For this review, take the finished solid that the model builds, in its own axes (mm). Face numbers are marked on the shaded views. A direction names the side the tool comes from. Round coordinates to 2 decimals unless told otherwise and drop trailing zeros. Write each loop counter-clockwise with the first axis right and the second up, starting at its lowest first coordinate (ties: lowest second). Pieces come first, ordered by that corner, then holes. Notation, with made-up numbers: M 6,58.25 L 20,58.25 A10 cw 20,76.25 Z; hole C -33.5,72.5 d3. An arc over 180 degrees is marked long. Answer in a Markdown table with one row per item.
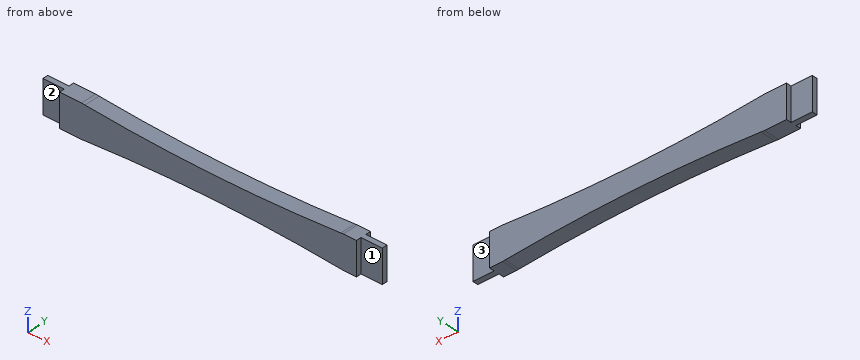
```python
from build123d import *

# Parameters (mm, degrees)
F0_W     = 406.4
F0_H     = 39.6875
F1_DEPTH = 9.525
F2_W     = 25.4
F2_H     = 6.35
F3_DEPTH = 39.6885
F5_DEPTH = 19.051


with BuildPart() as f1:
    # F0 (on Front) → F1 (new body, symmetric)
    with BuildSketch(Plane.XZ):
        Rectangle(F0_W, F0_H)
    extrude(amount=F1_DEPTH, both=True)

    # F2 (on face) → F3 (cut, through all)
    with BuildSketch(Plane.XY.offset(19.84375)):
        with Locations((190.5, -6.35)):
            Rectangle(F2_W, F2_H)
        with Locations((190.5, 6.35)):
            Rectangle(F2_W, F2_H)
        with Locations((-190.5, -6.35)):
            Rectangle(F2_W, F2_H)
        with Locations((-190.5, 6.35)):
            Rectangle(F2_W, F2_H)
    extrude(amount=-F3_DEPTH, mode=Mode.SUBTRACT)

    # F4 (on face) → F5 (cut, through all)
    with BuildSketch(Plane.XZ.offset(9.525)):
        with BuildLine():
            Line((162.1778154521, 19.84375), (-151.4870877189, 19.84375))
            ThreePointArc((-151.4870877189, 19.84375), (-149.3549908007, 19.6719963975), (-147.222705797, 19.5025938249))
            ThreePointArc((-147.222705797, 19.5025938249), (6.0616249582, 13.493882231), (159.3414767794, 19.6157851846))
            ThreePointArc((159.3414767794, 19.6157851846), (160.7596879137, 19.7292475425), (162.1778154521, 19.84375))
        make_face()
        with BuildLine():
            ThreePointArc((-147.222705797, -19.5025938249), (-149.3549908007, -19.6719963975), (-151.4870877189, -19.84375))
            Line((-151.4870877189, -19.84375), (162.1778154521, -19.84375))
            ThreePointArc((162.1778154521, -19.84375), (160.7596879137, -19.7292475425), (159.3414767794, -19.6157851846))
            ThreePointArc((159.3414767794, -19.6157851846), (6.0616249582, -13.493882231), (-147.222705797, -19.5025938249))
        make_face()
    extrude(amount=-F5_DEPTH, mode=Mode.SUBTRACT)


solid = f1.part
```
Q1. Take a section at D-D (x = 103). State the section outline as (y, z) points (3 decimals).
Found:
| item | result |
|---|---|
| outline | M -9.525,-15.953 L 9.525,-15.953 L 9.525,15.953 L -9.525,15.953 Z |
Q2. Insertion check: P1, Ø7, axis at y = -7.5, z = 5, coming from the +X side; P2, Ø12.5, axis at x = -190, z = 0, coming from the +Y side (3 decimals); P3, Ø7.5, axis at x = -192.5, z = -7, coming from the -Y side (3 decimals). Each pin has a flat end and moves straight along its axis. Give the tip position at first contact, or say it passes through.
Found:
| item | result |
|---|---|
| P1 | x = 177.8 |
| P2 | y = 3.175 |
| P3 | y = -3.175 |
Q3. Take a section at C-C (x = -100.5). State the section outline as (y, z) points (3 decimals).
Found:
| item | result |
|---|---|
| outline | M -9.525,-16.383 L 9.525,-16.383 L 9.525,16.383 L -9.525,16.383 Z |
Q4. Take a section at B-B (z = 0). State the section outline as (x, y) points (3 decimals).
Found:
| item | result |
|---|---|
| outline | M -203.2,-3.175 L -177.8,-3.175 L -177.8,-9.525 L 177.8,-9.525 L 177.8,-3.175 L 203.2,-3.175 L 203.2,3.175 L 177.8,3.175 L 177.8,9.525 L -177.8,9.525 L -177.8,3.175 L -203.2,3.175 Z |
Q5. Take a section at A-A (y = 0.25). State the section outline as (x, z) points, then the cut area to 3 significant figures.
Found:
| item | result |
|---|---|
| outline | M -203.2,-19.84 L -151.49,-19.84 A1939.9 cw -147.22,-19.5 A1939.9 cw 159.34,-19.62 A1939.9 cw 162.18,-19.84 L 203.2,-19.84 L 203.2,19.84 L 162.18,19.84 A1939.9 cw 159.34,19.62 A1939.9 cw -147.22,19.5 A1939.9 cw -151.49,19.84 L -203.2,19.84 Z |
| area | 13,500 mm² |
Q6. For probe 1 along X at (y, z) = (3.75, -11); probe 2 along Z at (x, y) = (-151, 4.5); probe 3 along Z at (x, y) = (64, 6), list the stretches that pass through material, from the lowest coordinate up.
Found:
| item | result |
|---|---|
| probe 1 | -177.8 to 177.8 |
| probe 2 | -19.8 to 19.8 |
| probe 3 | -14.38 to 14.38 |
Q7. Machinability: for the marked faces 1, 2 and 3, which of the approach directions +Z, -Z, +X, -X, +Y, -Y give a long, thin tool a straight path to every point of the face, cutting with its end or side? Answer none if there is none.
Found:
| item | result |
|---|---|
| face 1 | +Z, -Z, +X, -Y |
| face 2 | +Z, -Z, -X, -Y |
| face 3 | +Z, -Z, +X, +Y |
